Build history of the part. All positions in model axes, mm. A direction names the side the tool comes from. Round coordinates to 2 decimals unless told otherwise and drop trailing zeros. Loops run counter-clockwise (first coordinate to the right, second up) from the corner with the lowest first, then second, coordinate; pieces in that order, holes last.
from build123d import *

# Parameters (mm, degrees)
BOSS_EXTRUDE1_START       = -105
BOSS_EXTRUDE1_DEPTH       = 160
BOSS_EXTRUDE1_2_DEPTH     = 40
BOSS_EXTRUDE1_START_2     = -20
BOSS_EXTRUDE1_3_OUTLINE_W = 48
BOSS_EXTRUDE1_3_OUTLINE_H = 147
BOSS_EXTRUDE1_3_DEPTH     = 20
BOSS_EXTRUDE1_START_3     = 42.132444372
BOSS_EXTRUDE1_4_OUTLINE_W = 52
BOSS_EXTRUDE1_4_OUTLINE_H = 116
BOSS_EXTRUDE1_4_DEPTH     = 19.867555628
BOSS_EXTRUDE1_START_4     = 80.434666527
BOSS_EXTRUDE1_5_OUTLINE_W = 52
BOSS_EXTRUDE1_5_OUTLINE_H = 117
BOSS_EXTRUDE1_5_DEPTH     = 20.565333473
SKETCH2_W                 = 21.285197014
SKETCH2_H                 = 16.738844255
BOSS_EXTRUDE2_DEPTH       = 10
SKETCH3_R                 = 75
CUT_EXTRUDE1_DEPTH        = 95


with BuildPart() as part:
    # Boss-Extrude1: read off the stored shape, not the designer's step
    # Boss-Extrude1 outline → Boss-Extrude1 (new body)
    with BuildSketch(Plane.XY.offset(BOSS_EXTRUDE1_START)):
        Polygon((65, 0), (40, 29.793839815), (15, 0), align=None)
    extrude(amount=BOSS_EXTRUDE1_DEPTH)

    # Boss-Extrude1 2 outline → Boss-Extrude1 2 (add)
    with BuildSketch(Plane.YZ):
        Polygon((0, -50), (29.793839815, -25), (0, 0), align=None)
    extrude(amount=BOSS_EXTRUDE1_2_DEPTH)

    # Boss-Extrude1 3 outline → Boss-Extrude1 3 (cut)
    with BuildSketch(Plane(origin=(0, 0, 0), x_dir=(0.6427876096865404, 0.7660444431189772, 0), z_dir=(0.7660444431189772, -0.6427876096865403, 0)).offset(BOSS_EXTRUDE1_START_2)):
        with Locations((22, -24.5)):
            Rectangle(BOSS_EXTRUDE1_3_OUTLINE_W, BOSS_EXTRUDE1_3_OUTLINE_H)
    extrude(amount=BOSS_EXTRUDE1_3_DEPTH, mode=Mode.SUBTRACT)

    # Boss-Extrude1 4 outline → Boss-Extrude1 4 (cut)
    with BuildSketch(Plane(origin=(0, 0, 0), x_dir=(1, 0, 0), z_dir=(0, 0.6427876096865403, 0.7660444431189772)).offset(BOSS_EXTRUDE1_START_3)):
        with Locations((40, 21)):
            Rectangle(BOSS_EXTRUDE1_4_OUTLINE_W, BOSS_EXTRUDE1_4_OUTLINE_H)
    extrude(amount=BOSS_EXTRUDE1_4_DEPTH, mode=Mode.SUBTRACT)

    # Boss-Extrude1 5 outline → Boss-Extrude1 5 (cut)
    with BuildSketch(Plane(origin=(0, 0, 0), x_dir=(1, 0, 0), z_dir=(0, 0.6427876096865403, -0.7660444431189772)).offset(BOSS_EXTRUDE1_START_4)):
        with Locations((40, 10.5)):
            Rectangle(BOSS_EXTRUDE1_5_OUTLINE_W, BOSS_EXTRUDE1_5_OUTLINE_H)
    extrude(amount=BOSS_EXTRUDE1_5_DEPTH, mode=Mode.SUBTRACT)

    # Sketch2 → Boss-Extrude2 (add)
    with BuildSketch(Plane.XZ):
        with Locations((0.693235287, -25.516630996)):
            Rectangle(SKETCH2_W, SKETCH2_H)
    extrude(amount=-BOSS_EXTRUDE2_DEPTH)

    # Mirror8: part across plane


with BuildPart() as part_1:
    add(part.part)
    add(part.part.mirror(Plane(origin=(-9.94936322, 10, -17.147208868), x_dir=(0, 0, 1), z_dir=(-1, 0, 0))))

    # Sketch3 → Cut-Extrude1 (cut, symmetric)
    with BuildSketch(Plane.XY):
        with Locations((-9.94936322, 85)):
            Circle(SKETCH3_R)
    extrude(amount=CUT_EXTRUDE1_DEPTH, both=True, mode=Mode.SUBTRACT)


solid = part_1.part
(1) Slice it at C-C on x = 26. List the corners of the cut face in (y, z).
Responses:
outline: (0, -105) - (13.11, -94) - (13.11, -39) - (19.18, -33.91) - (19.18, -16.09) - (13.11, -11) - (13.11, 44) - (0, 55) - close
(2) Pin check, flat tips, straight feed: P1, Ø8, axis at y = 20.5, z = -76, coming from the -X side; P2, Ø5, axis at x = -13.5, y = 4.5, coming from the -Z side; P3, Ø4, axis at y = 20.5, z = 21.5, coming from the +X side. Stop position of each tip, or through.
Responses:
P1: stops at x = -71.05
P2: stops at z = -33.89
P3: stops at x = 49.48
(3) Slice it at B-B on y = 15. List the corners of the cut face in (x, z), plus the area to 3 significant figures.
Responses:
outline: (-72.31, -92.41) - (-47.49, -92.41) - (-47.49, -37.41) - (-36.88, -37.41) - (-36.88, -12.59) - (-47.49, -12.59) - (-47.49, 42.41) - (-72.31, 42.41) - close; (16.98, -37.41) - (27.59, -37.41) - (27.59, -92.41) - (52.41, -92.41) - (52.41, 42.41) - (27.59, 42.41) - (27.59, -12.59) - (16.98, -12.59) - close
area: 7,220 mm2
(4) Which spindle directions (+Z, -Z, +X, -X, +Y, -Y) get a long thin tool onto all of the face, cutting with end or side? Do faces 5 (the face through (16.003, 9.615, -8.068)), 6 (the face through (-46.447, 13.763, -66.655)), 7 (the face through (8.98, 10.7, -24.65)). Say none if no direction does.
Responses:
face 5: +Z, +Y
face 6: -Z, +Y
face 7: +Y
(5) Slice it at A-A on z = 12.5. List the corners of the cut face in (x, y).
Responses:
outline: (-84.9, 0) - (-34.9, 0) - (-57.68, 27.15) arc R75 cw to (-60.25, 29.37) - close; (15, 0) - (65, 0) - (40.35, 29.37) arc R75 cw to (37.78, 27.15) - close
(6) Probe line 1 (X direction, y = 3, z = -91); line 2 (X direction, y = 25.25, z = -73.5); line 3 (Y direction, x = -64.5, z = -33). List the from-to ranges inside material, lowest first.
Responses:
line 1: x = -82.38 to -37.42, 17.52 to 62.48
line 2: x = -63.71 to -56.09, 36.19 to 43.81
line 3: y = 0 to 24.31
(7) Slice it at D-D on z = -5. List the corners of the cut face in (x, y), plus the area to 3 significant figures.
Responses:
outline: (-84.9, 0) - (-19.9, 0) - (-24.9, 5.96) - (-39.9, 5.96) - (-57.68, 27.15) arc R75 cw to (-60.25, 29.37) - close; (0, 0) - (65, 0) - (40.35, 29.37) arc R75 cw to (37.78, 27.15) - (20, 5.96) - (5, 5.96) - close
area: 1,670 mm2
(8) Pull direction X, two halves, no side cores. Call faces 1 (the face through (26.549, 13.763, 15.566)), 2 (the face through (52.85, 14.48, -26.12)), 3 (the face through (-35.901, 8.483, -42.882)), 4 (the face through (-9, 0, -24)): +X half, -X half, draft (parallel to the pull), parting line (faces both ways), or undercut.
Responses:
face 1: undercut
face 2: +X half
face 3: undercut
face 4: draft
